For this review, take the finished solid that the model builds, in its own axes (mm). Give positions to 0.01 mm unless a question says otherwise; leave off trailing zeros. Order: outer loops, then holes, each group sorted by start corner. A loop starts at its lowest first (then second) coordinate and runs counter-clockwise, first axis right, second up. Notation, with made-up numbers: (-0.5, 14.25) - (36.5, 14.25) arc R17 ccw to (36.5, 22.25) - close; hole circle Ø1 at (3, -16). An arc over 180 degrees is marked (long way). Use a Markdown table: item, result. Add a question column.
1) We need section A-A on x = 12. Write out the cut boundary in (y, z).
2) Clearance check with a flat-ended pin moving along its axis: P1, Ø4.5, axis at x = 94, z = -54, coming from the -Y side. State where the tip first meets the part, or that it passes through.
3) Mouldability with a two-part tool opening along Z and no side actions: class faces 1 (the face through (4, 1.588, 2)), 2 (the face through (-192.697, 0.805, 9.736)) as released by +Z, released by -Z, zero draft, split by the parting line, or undercut.
4) Wall thickness on L1, parallel to X at y = 1, z = 46.75 (3 decimals); L2, parallel to Z at x = 94, y = 1; L3, parallel to X at y = 0.15, z = -47.5 (3 decimals): over which ranges is each line inside the solid? List them lowest first.
Autodesk Inventor part; units mm, degrees
ref_plane "YZ Plane" through (0, 0, 0) normal (1, 0, 0) x (0, 1, 0)
ref_plane "XZ Plane" through (0, 0, 0) normal (0, 1, 0) x (-1, 0, 0)
ref_plane "XY Plane" through (0, 0, 0) normal (0, 0, 1) x (1, 0, 0)
sketch "Sketch1" plane through (0, 0, 0) normal (0, 1, 0) x (-1, 0, 0)
  line L0 (-305.435, 114.3) -> (305.435, 114.3)
  line L1 (305.435, 114.3) -> (305.435, -114.3)
  line L2 (305.435, -114.3) -> (-305.435, -114.3)
  line L3 (-305.435, -114.3) -> (-305.435, 114.3)
  line L4 (-305.435, 114.3) -> (305.435, -114.3) construction
  line L5 (305.435, 114.3) -> (-305.435, -114.3) construction
  point P0 (0, 0)
  dimension "d0" = 610.87
  dimension "d1" = 228.6
extrude "Extrusion1" add sketch "Sketch1" along normal blind 1.5875
sketch "Sketch3" plane through (0, 1.5875, 0) normal (0, 1, 0) x (1, 0, 0)
  circle A0 centre (-180, 0) radius 93.5 construction
  circle A1 centre (-180, 93.5) radius 4
  circle A2 centre (-226.75, 80.9734) radius 4
  circle A3 centre (-260.9734, 46.75) radius 4
  circle A4 centre (-273.5, 0) radius 4
  circle A5 centre (-260.9734, -46.75) radius 4
  circle A6 centre (-226.75, -80.9734) radius 4
  circle A7 centre (-180, -93.5) radius 4
  circle A8 centre (-133.25, -80.9734) radius 4
  circle A9 centre (-99.0266, -46.75) radius 4
  circle A10 centre (-86.5, 0) radius 4
  circle A11 centre (-99.0266, 46.75) radius 4
  circle A12 centre (-133.25, 80.9734) radius 4
  circle A13 centre (-180, 0) radius 16
  point P0 (0, 0)
  dimension "d5" = 187
  dimension "d6" = 180
  dimension "d7" = 8
  dimension "d10" = 360
  dimension "d12" = 32
extrude "Extrusion2" cut sketch "Sketch3" against normal through all
sketch "Sketch4" plane through (0, 1.5875, 0) normal (0, 1, 0) x (1, 0, 0)
  circle A0 centre (-180, 0) radius 16 construction
  circle A1 centre (32, 0) radius 7 construction
  circle A2 centre (-24, 48) radius 2.5 construction
  circle A3 centre (-30, 54) radius 2
  circle A4 centre (-30, 42) radius 2
  circle A5 centre (-18, 42) radius 2
  circle A6 centre (-18, 54) radius 2
  line L0 (32, 7) -> (32, -7) construction
  line L1 (25, 0) -> (39, 0) construction
  circle A7 centre (94, 54) radius 2
  circle A8 centre (94, 42) radius 2
  circle A9 centre (82, 42) radius 2
  circle A10 centre (82, 54) radius 2
  circle A11 centre (-30, -54) radius 2
  circle A12 centre (-30, -42) radius 2
  circle A13 centre (-18, -42) radius 2
  circle A14 centre (-18, -54) radius 2
  circle A15 centre (94, -54) radius 2
  circle A16 centre (94, -42) radius 2
  circle A17 centre (82, -42) radius 2
  circle A18 centre (82, -54) radius 2
  circle A19 centre (52, 0) radius 7
  circle A20 centre (12, 0) radius 7
  point P0 (0, 0)
  dimension "d22" = 14
  dimension "d23" = 212
  dimension "d24" = 5
  dimension "d25" = 56
  dimension "d26" = 48
  dimension "d27" = 4
  dimension "d28" = 6
  dimension "d29" = 6
  dimension "d34" = 360
  dimension "d36" = 14
  dimension "d37" = 20
  dimension "d38" = 14
  dimension "d40" = 20
extrude "Extrusion3" cut sketch "Sketch4" against normal through all
properties part number "ChassisTop V2"
Checked values:
| question | item | result |
|---|---|---|
| 1 | outline | (0, -114.3) - (1.59, -114.3) - (1.59, -7) - (0, -7) - close; (0, 7) - (1.59, 7) - (1.59, 114.3) - (0, 114.3) - close |
| 2 | P1 | y = 0 |
| 3 | face 1 | zero draft |
| 3 | face 2 | undercut |
| 4 | L1 | -305.435 to -264.973, -256.973 to -103.027, -95.027 to 305.435 |
| 4 | L2 | -114.3 to -56, -52 to -44, -40 to 40, 44 to 52, 56 to 114.3 |
| 4 | L3 | -305.435 to -264.902, -257.044 to -102.956, -95.098 to 305.435 |
